Work out the finished part from the listing and answer in its coordinate system (mm). Face numbers are marked on the shaded views. Round coordinates to 2 decimals unless told otherwise and drop trailing zeros. Write each loop counter-clockwise with the first axis right and the second up, starting at its lowest first coordinate (ties: lowest second). Pieces come first, ordered by that corner, then holes.
1. Find section A-A (z = 5). Write down the section's boundary in (x, y).
2. Flat-ended cylindrical pins translate along their axes: pin 1 Ø4 at (y, z) = (-42, 7.5) entering from +X; pin 2 Ø4 at (x, z) = (-10, 7.5) entering from -Y; pin 3 Ø3 at (y, z) = (-18, 9.5) entering from -X. Find the tip coordinate at first contact, or state that the pin passes through.
3. Find section B-B (x = -17). Write down the section's boundary in (y, z).
4. Find section D-D (y = -53.5). Write down the section's boundary in (x, z).
5. Straight lines are drawn through the part: probe 1 along Y at (x, z) = (-14, 9.25); probe 2 along Y at (x, z) = (-12, 3.5); probe 3 along Y at (x, z) = (-8, 10.5). For each, find the intervals that lie inside material, in ascending order.
6. Find section C-C (x = -2.5). Write down the section's boundary in (y, z), and give its area (3 significant figures).
7. Determine the mould class of the marked faces 1, 2, 3 and 4 for opening direction Y: pulls with the +Y half, pulls with the -Y half, needs draft (parallel to the pull), parting line crosses it, or undercut.
```python
from build123d import *

# Parameters (mm, degrees)
RESSALTO_EXTRUS_O1_DEPTH = 11.849977


with BuildPart() as part:
    # Esboço1 → Ressalto-extrusão1 (new body)
    with BuildSketch(Plane.XY):
        with BuildLine():
            ThreePointArc((-10.685745363, -67.703603991), (-26.769323244, -33.991425444), (2.462180193, -10.738217779))
            Line((2.462180193, -10.738217779), (2.462180193, -0.672237217))
            Line((2.462180193, -0.672237217), (2.462180193, 19.360753065))
            ThreePointArc((2.462180193, 19.360753065), (-0.537819807, 22.360753065), (-3.537819807, 19.360753065))
            Line((-3.537819807, 19.360753065), (-3.478607435, 18.767652629))
            Line((-3.478607435, 18.767652629), (-0.816088481, -7.901455538))
            ThreePointArc((-0.816088481, -7.901455538), (-26.821074104, -25.523388901), (-26.291187743, -56.932162089))
            Line((-26.291187743, -56.932162089), (-31.663381791, -61.605561148))
            ThreePointArc((-31.663381791, -61.605561148), (-24.444874339, -70.335690922), (-15.068387215, -76.692066062))
            Line((-15.068387215, -76.692066062), (-10.685745363, -67.703603991))
        make_face()
    extrude(amount=RESSALTO_EXTRUS_O1_DEPTH)


solid = part.part
```
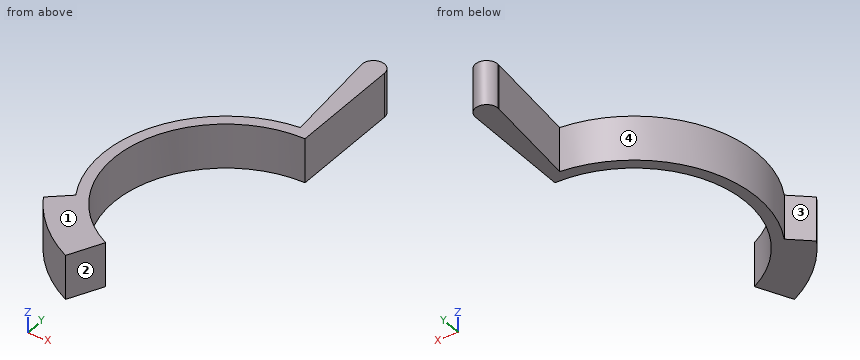
Worked answers:
1. outline: (-31.66, -61.61) arc R40 ccw to (-15.07, -76.69) - (-10.69, -67.7) arc R30 cw to (2.46, -10.74) - (2.46, 19.36) arc R3 ccw to (-3.54, 19.36) - (-0.82, -7.9) arc R33 ccw to (-26.29, -56.93) - close
2. pin 1: stops at x = -27.36
2. pin 2: stops at y = -70.4
2. pin 3: stops at x = -22.8
3. outline: (-75.68, 0) - (-63.57, 0) - (-63.57, 11.85) - (-75.68, 11.85) - close; (-17.91, 0) - (-14.09, 0) - (-14.09, 11.85) - (-17.91, 11.85) - close
4. outline: (-27.97, 0) - (-24.69, 0) - (-24.69, 11.85) - (-27.97, 11.85) - close
5. probe 1: y = -74.5 to -65.82, -15.66 to -12.14
5. probe 2: y = -70.4 to -67.02, -14.45 to -11.08
5. probe 3: y = -12.62 to -9.44
6. outline: (-11.15, 0) - (-8.11, 0) - (-8.11, 11.85) - (-11.15, 11.85) - close; (8.97, 0) - (21.63, 0) - (21.63, 11.85) - (8.97, 11.85) - close
6. area: 186 mm2
7. face 1: needs draft
7. face 2: pulls with the -Y half
7. face 3: undercut
7. face 4: undercut
